Part model, mm, in its own coordinate system. Give positions to 0.01 mm unless a question says otherwise; leave off trailing zeros. Order: outer loops, then holes, each group sorted by start corner. A loop starts at its lowest first (then second) coordinate and runs counter-clockwise, first axis right, second up. Notation, with made-up numbers: (-6, 26) -> (22, 26) arc R23 ccw to (22, 40) -> close; hole circle Ø2 at (17.5, 74.5). An arc over 180 degrees is marked (long way). Write item = value, one per line. Start each with the question number.
(1) Saw through at D-D, the plane z = -604. List the corners of the cut face in (x, y), then the cut area to 3 significant figures.
(2) Saw through at A-A, the plane z = -624. List the corners of the cut face in (x, y), then the cut area to 3 significant figures.
(3) Saw through at B-B, the plane y = -60. List the corners of the cut face in (x, z), then the cut area to 3 significant figures.
(4) Probe line 1 along Z through (x, y) = (-1.9, -55); line 2 along Y through (x, z) = (-1.85, -650); line 3 along Y through (x, z) = (-1.2, -602.5). List the from-to ranges inside material, lowest first. Write a range as from..to.
(5) Saw through at C-C, the plane x = -1.6. List the corners of the cut face in (y, z).
(6) Flat gauge pins, fed straight in: pin 1 (1.8 mm diameter, centred on y = -75.33, z = -609.52, fed in from -X); pin 2 (0.6 mm diameter, centred on x = -0.5, y = -58.5, fed in from +Z). Where does each tip first touch, or does it go through?
Autodesk Inventor part; units mm, degrees
ref_plane "YZ Plane" through (0, 0, 0) normal (1, 0, 0) x (0, 1, 0)
ref_plane "XZ Plane" through (0, 0, 0) normal (0, 1, 0) x (-1, 0, 0)
ref_plane "XY Plane" through (0, 0, 0) normal (0, 0, 1) x (1, 0, 0)
sketch "スケッチ1" plane through (0, 0, 0) normal (1, 0, 0) x (0, 1, 0)
  line L0 (-65.3332, -639.5232) -> (-65.3332, 668.4768)
  line L1 (-65.3332, -537.5232) -> (339.6668, -537.5232)
  line L2 (339.6668, -537.5232) -> (339.6668, -517.5232)
  line L3 (339.6668, -517.5232) -> (-65.3332, -517.5232)
  line L4 (-65.3332, -517.5232) -> (-65.3332, -537.5232)
  circle A0 centre (-30.1532, -490.5232) radius 21
  circle A1 centre (-30.1532, -448.5232) radius 16
  circle A2 centre (-30.1532, -448.5232) radius 13.68
  line L5 (-85.3332, -639.5232) -> (-65.3332, -639.5232)
  line L6 (-85.3332, -639.5232) -> (-65.3332, -639.5232)
  line L7 (-85.3332, -639.5232) -> (398.6668, -639.5232)
  line L8 (398.6668, -639.5232) -> (398.6668, -659.5232)
  line L9 (398.6668, -659.5232) -> (-85.3332, -659.5232)
  line L10 (-85.3332, -659.5232) -> (-85.3332, -639.5232)
  line L11 (-10.1532, 668.4768) -> (9.0226, 674.1594)
  line L12 (9.0226, 674.1594) -> (394.8699, -627.872)
  line L13 (394.8699, -627.872) -> (375.6942, -633.5546)
  line L14 (375.6942, -633.5546) -> (-10.1532, 668.4768)
  line L15 (-85.3332, 668.4768) -> (-85.3332, -639.5232)
  line L16 (-85.3332, -432.5232) -> (-30.1532, -432.5232)
  line L17 (-9.1532, -490.5232) -> (-9.1532, -537.5232)
  line L18 (-9.1532, -490.5232) -> (-9.1532, -432.5232)
  line L19 (-9.1532, -432.5232) -> (-30.1532, -432.5232)
  circle A3 centre (-75.3332, -444.5232) radius 1.5
  circle A4 centre (-75.3332, -454.5232) radius 1.5
  line L20 (-30.1532, -464.5232) -> (-85.3332, -464.5232)
  circle A5 centre (-55.3332, -527.5232) radius 1.5
  circle A6 centre (-35.3332, -527.5232) radius 1.5
  line L21 (-65.3332, -537.5232) -> (-85.3332, -537.5232)
  circle A7 centre (-75.3332, -527.5232) radius 1.5
  circle A8 centre (-75.3332, -507.5232) radius 1.5
  circle A9 centre (-30.1532, 652.4768) radius 16
  line L22 (-65.3332, 668.4768) -> (-85.3332, 668.4768)
  line L23 (-85.3332, 668.4768) -> (-30.1532, 668.4768)
  line L24 (-30.1532, 636.4768) -> (-85.3332, 636.4768)
  line L25 (-30.1532, 668.4768) -> (-10.1532, 668.4768)
  circle A10 centre (-30.1532, 652.4768) radius 7.5
  line L26 (-30.1532, 636.4768) -> (-0.6702, 636.4768)
  circle A11 centre (-75.3332, 656.4768) radius 1.5
  circle A12 centre (-75.3332, 646.4768) radius 1.5
  circle A13 centre (2.276, 661.7302) radius 1.5
  circle A14 centre (5.1173, 652.1424) radius 1.5
  line L27 (-0.6702, 636.4768) -> (18.5055, 642.1594)
  line L28 (-65.3332, -599.5232) -> (-45.3332, -639.5232)
  line L29 (-45.3332, -639.5232) -> (-45.3332, -659.5232)
  line L30 (-65.3332, -599.5232) -> (-85.3332, -599.5232)
  circle A15 centre (-75.3332, -629.5232) radius 1.5
  circle A16 centre (-75.3332, -619.5232) radius 1.5
  circle A17 centre (-75.3332, -609.5232) radius 1.5
  circle A18 centre (-75.3332, -649.5232) radius 1.5
  circle A19 centre (-65.3332, -649.5232) radius 1.5
  circle A20 centre (-55.3332, -649.5232) radius 1.5
  line L31 (-85.3332, -639.5232) -> (-85.3332, -599.5232)
  line L32 (368.6668, -639.5232) -> (368.6668, -659.5232)
  line L33 (367.1703, -604.7911) -> (386.346, -599.1085)
  line L34 (375.6942, -633.5546) -> (377.4629, -639.5232)
  line L35 (394.8699, -627.872) -> (398.6668, -639.5232)
  circle A21 centre (378.6668, -649.5232) radius 1.5
  circle A22 centre (388.6668, -649.5232) radius 1.5
  circle A23 centre (382.4407, -621.1255) radius 1.5
  circle A24 centre (379.5994, -611.5376) radius 1.5
  circle A25 centre (319.6668, -527.5232) radius 1.5
  circle A26 centre (329.6668, -527.5232) radius 1.5
  line L36 (339.6668, -517.5232) -> (341.3091, -517.5232)
  line L37 (339.6668, -537.5232) -> (347.236, -537.5232)
  line L38 (341.3091, -517.5232) -> (362.1688, -517.5232)
  circle A27 centre (354.5961, -527.1644) radius 1.5
  circle A28 centre (357.4374, -536.7523) radius 1.5
  line L39 (350.6908, -549.1815) -> (369.8665, -543.4989)
  line L40 (309.6668, -517.5232) -> (309.6668, -537.5232)
  line L41 (-50.3332, -659.5232) -> (-50.3332, -640.7035)
  line L42 (-50.3332, -640.7035) -> (-68.4233, -604.5232)
  line L43 (-68.4233, -604.5232) -> (-80.3332, -604.5232)
  line L44 (-80.3332, -604.5232) -> (-80.3332, -639.5232)
  point P0 (0, 0)
  point P1 (-388.3332, -207.1898)
  point P2 (-65.3332, -517.5232)
  point P3 (385.282, -630.7133)
  point P4 (-50.9233, -639.5232)
  point P5 (-65.3332, -610.7035)
  dimension "d1" = 42
  dimension "d0" = 20
  dimension "d2" = 32
  dimension "d3" = 27.36
  dimension "d4" = 35.18
  dimension "d5" = 35.18
  dimension "d6" = 27
  dimension "d7" = 42
  dimension "d8" = 191
  dimension "d9" = 20
  dimension "d10" = 484
  dimension "d11" = 3
  dimension "d12" = 3
  dimension "d13" = 10
  dimension "d14" = 10
  dimension "d15" = 10
  dimension "d16" = 10
  dimension "d17" = 3
  dimension "d18" = 3
  dimension "d19" = 10
  dimension "d20" = 20
  dimension "d21" = 10
  dimension "d22" = 10
  dimension "d23" = 3
  dimension "d24" = 3
  dimension "d25" = 10
  dimension "d26" = 20
  dimension "d27" = 10
  dimension "d28" = 10
  dimension "d29" = 20
  dimension "d30" = 32
  dimension "d31" = 35.18
  dimension "d32" = 20
  dimension "d33" = 1358
  dimension "d34" = 91.543
  dimension "d35" = 405
  dimension "d36" = 15
  dimension "d37" = 3
  dimension "d38" = 3
  dimension "d39" = 10
  dimension "d40" = 10
  dimension "d41" = 10
  dimension "d42" = 10
  dimension "d43" = 3
  dimension "d44" = 3
  dimension "d45" = 10
  dimension "d46" = 10
  dimension "d47" = 10
  dimension "d48" = 10
  dimension "d49" = 40
  dimension "d50" = 3
  dimension "d51" = 3
  dimension "d52" = 3
  dimension "d53" = 3
  dimension "d54" = 3
  dimension "d55" = 3
  dimension "d56" = 10
  dimension "d57" = 10
  dimension "d58" = 10
  dimension "d59" = 10
  dimension "d60" = 10
  dimension "d61" = 10
  dimension "d62" = 10
  dimension "d63" = 10
  dimension "d64" = 10
extrude "押し出し1" add sketch "スケッチ1" against normal blind 2 contours L28 L7 L42 L0 | L0 L42 L43 L44 L5 L15 L30 | L42 L7 L0 | L0 L5 L44 L43 L42 | L29 L9 L41 L42 L7 | L7 L42 L41 L9 L10 L5
extrude "押し出し2" cut sketch "スケッチ1" against normal blind 2 contours L42 L7 L0
fillet "フィレット1" radius 2 8 edges at (-1, -85.3332, -599.5232) (-1, -65.3332, -599.5232) (-1, -65.3332, -610.7035) (-1, -65.3332, -639.5232) (-1, -50.9233, -639.5232) (-1, -45.3332, -639.5232) (-1, -45.3332, -659.5232) (-1, -85.3332, -659.5232)
equation "\"d14\" = d15"
equation "\"d21\" = d19"
equation "\"d22\" = d19"
equation "\"d27\" = d25"
equation "\"d28\" = d25"
equation "\"d31\" = d4"
equation "\"d41\" = d39"
equation "\"d42\" = d39"
equation "\"d46\" = d45"
equation "\"d47\" = d45"
equation "\"d48\" = d45"
equation "\"d57\" = d56"
equation "\"d58\" = d56"
equation "\"d59\" = d56"
equation "\"d60\" = d56"
equation "\"d61\" = d56"
equation "\"d62\" = d56"
equation "\"d63\" = d56"
equation "\"d64\" = d62"
properties part number "dribl-v1-Plate-9" material "アルミニウム 6061"
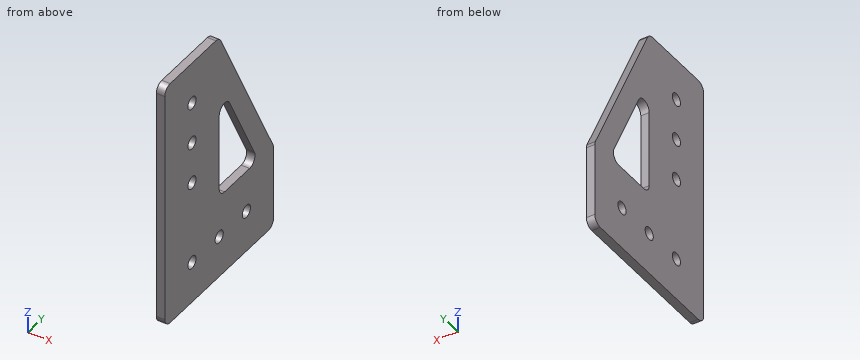
Results list:
q1.outline = (-2, -85.33) -> (0, -85.33) -> (0, -63.09) -> (-2, -63.09) -> close
q1.area = 44.5 mm^2
q2.outline = (-2, -85.33) -> (0, -85.33) -> (0, -65.33) -> (-2, -65.33) -> close; (-2, -58.68) -> (0, -58.68) -> (0, -53.09) -> (-2, -53.09) -> close
q2.area = 51.2 mm^2
q3.outline = (-2, -659.52) -> (0, -659.52) -> (0, -639.52) -> (-2, -639.52) -> close; (-2, -621.37) -> (0, -621.37) -> (0, -610.19) -> (-2, -610.19) -> close
q3.area = 62.4 mm^2
q4.line_1 = -659.52..-650.99, -648.06..-639.52, -631.37..-620.19
q4.line_2 = -85.33..-76.76, -73.91..-66.76, -63.91..-56.76, -53.91..-45.33
q4.line_3 = -85.33..-63.84
q5.outline = (-85.33, -657.52) arc R2 ccw to (-83.33, -659.52) -> (-47.33, -659.52) arc R2 ccw to (-45.33, -657.52) -> (-45.33, -640) arc R2 ccw to (-45.54, -639.1) -> (-64.78, -600.63) arc R2 ccw to (-66.57, -599.52) -> (-83.33, -599.52) arc R2 ccw to (-85.33, -601.52) -> close; hole circle Ø3 at (-75.33, -649.52); hole circle Ø3 at (-75.33, -629.52); hole circle Ø3 at (-75.33, -619.52); hole circle Ø3 at (-75.33, -609.52); hole circle Ø3 at (-65.33, -649.52); hole (-65.33, -637.52) arc R2 ccw to (-63.33, -639.52) -> (-54.16, -639.52) arc R2 ccw to (-52.37, -636.63) -> (-61.54, -618.28) arc R2 ccw to (-65.33, -619.18) -> close; hole circle Ø3 at (-55.33, -649.52)
q6.pin_1 = through
q6.pin_2 = -612.59
